Verification items for the finished model (mm, model axes). Face numbers are marked on the shaded views. A direction names the side the tool comes from. Give positions to 0.01 mm unless a question says otherwise; leave off trailing zeros. Write each loop counter-clockwise with the first axis right and the second up, starting at its lowest first coordinate (ties: lowest second). Pieces come first, ordered by that corner, then holes. Notation, with made-up numbers: (81, 51) - (110, 51) arc R28 cw to (110, 83) - close; hole circle Ø4 at (49.5, 42.25). An arc over 180 degrees is marked (long way). Answer as a JSON object with one key per item and string values. Group by question number.
Item 1: Tool access check on the marked faces 1, 2, 3, 4 and 5. Record the directions out of +Z, -Z, +X, -X, +Y, -Y that give a thin tool (end or side, any length) a straight path to the whole face; none if there is none.
Item 2: Sectioned sample at C-C, the plane z = 84. Record the boundary of the cut face in (x, y).
Item 3: Sectioned sample at A-A, the plane y = -46. Record the boundary of the cut face in (x, z), and give its area (3 significant figures).
Item 4: Go/stop test with flat-tipped pins: pin 1 (7.5 mm diameter, centred on x = 35, y = -50, fed in from -Z); pin 2 (5 mm diameter, centred on x = -6.5, z = 36.5, fed in from -Y); pin 3 (3 mm diameter, centred on x = -19.5, y = -58.5, fed in from +Z). Record where each tip stops, or that it passes through.
Item 5: Sectioned sample at D-D, the plane y = -6. Record the boundary of the cut face in (x, z).
Item 6: Draft check along X on the marked faces 6, 7, 8 and 9. Enter one of: +X half, -X half, draft (parallel to the pull), parting line (faces both ways), or undercut.
Item 7: Scan lines: line 1 along X through (y, z) = (-55, 15); line 2 along X through (y, z) = (-12.75, 84); line 3 along Z through (x, y) = (-1, -22.5). Record each from-to range of solid material in increasing order. Write a range as [from, to].
Item 8: Sectioned sample at B-B, the plane x = -3.5. Record the boundary of the cut face in (y, z), and give its area (3 significant figures).
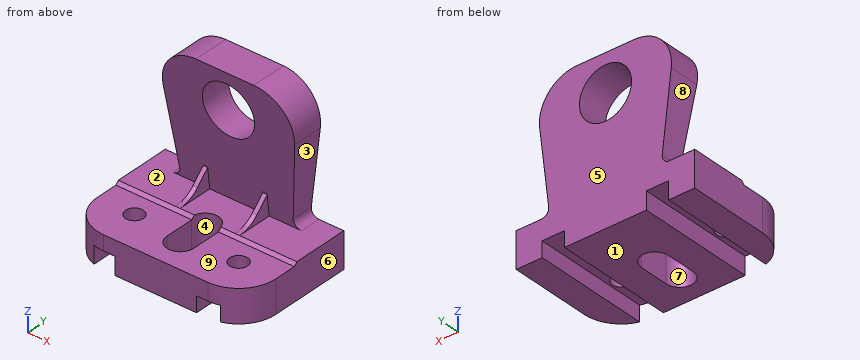
```python
from build123d import *

# Parameters (mm, degrees)
F1_DEPTH      = 60
F2_W          = 15
F2_H          = 11.9018135592
F2_H_2        = 10.3764180094
F3_DEPTH      = 80.001
F5_DEPTH      = 80.001
F6_W          = 3
F6_H          = 15
F7_DEPTH      = 40
F9_DEPTH      = 60.001
F9_DEPTH_BACK = 60.001
F11_D         = 12.1
F13_DEPTH     = 109.001
F15_D         = 35
F16_R         = 25
F17_SIZE      = 1.99999


# Not quite as in the source:
# - a fillet or chamfer is up to 0.001 mm smaller than in the source, because OpenCascade refuses the exact size


with BuildPart() as f1:
    # F0 (on Right) → F1 (new body, symmetric)
    with BuildSketch(Plane.YZ):
        Polygon((-80, 0), (0, 0), (0, 109), (-24, 109), (-14.0000553612, 24), (-40, 24), (-40, 22), (-80, 22), align=None)
    extrude(amount=F1_DEPTH, both=True)

    # F2 (on Front) → F3 (cut, through all)
    with BuildSketch(Plane.XZ):
        with Locations((-35, 5.9509067796)):
            Rectangle(F2_W, F2_H)
        with Locations((35, 5.1882090047)):
            Rectangle(F2_W, F2_H_2)
    extrude(amount=F3_DEPTH, mode=Mode.SUBTRACT)

    # F4 (on Front) → F5 (cut, through all)
    with BuildSketch(Plane.XZ):
        with BuildLine():
            ThreePointArc((-43.1227148243, 24), (-39.3863385559, 25.6774268435), (-38.1569614274, 29.5842030478))
            Line((-38.1569614274, 29.5842030478), (-44.2151375018, 81.0789847612))
            ThreePointArc((-44.2151375018, 81.0789847612), (-38.0682518594, 100.6128657827), (-19.3863705172, 109))
            Line((-19.3863705172, 109), (0, 109))
            Line((0, 109), (19.3863705172, 109))
            ThreePointArc((19.3863705172, 109), (38.0682518594, 100.6128657827), (44.2151375018, 81.0789847612))
            Line((44.2151375018, 81.0789847612), (38.1569614274, 29.5842030478))
            ThreePointArc((38.1569614274, 29.5842030478), (39.3863385559, 25.6774268435), (43.1227148243, 24))
            Line((43.1227148243, 24), (60, 24))
            Line((60, 24), (60, 136.873498559))
            Line((60, 136.873498559), (-60, 136.873498559))
            Line((-60, 136.873498559), (-60, 24))
            Line((-60, 24), (-43.1227148243, 24))
        make_face()
    extrude(amount=F5_DEPTH, mode=Mode.SUBTRACT)

    # F6 (on Front) → F7 (join, through all)
    with BuildSketch(Plane.XZ):
        with Locations((-20, 31.5)):
            Rectangle(F6_W, F6_H)
        with Locations((20, 31.5)):
            Rectangle(F6_W, F6_H)
    extrude(amount=F7_DEPTH)

    # F8 (on Right) → F9 (cut, two sides)
    with BuildSketch(Plane.YZ) as f9_sk:
        with BuildLine():
            Line((-23.8578643763, 29.8578643763), (-15.6543285765, 38.061400176))
            Line((-15.6543285765, 38.061400176), (-16.3282091593, 43.7894168409))
            Line((-16.3282091593, 43.7894168409), (-43.991163373, 43.7894168409))
            Line((-43.991163373, 43.7894168409), (-43.991163373, 24))
            Line((-43.991163373, 24), (-38, 24))
            ThreePointArc((-38, 24), (-30.3463313527, 25.5224093498), (-23.8578643763, 29.8578643763))
        make_face()
    extrude(amount=-F9_DEPTH, mode=Mode.SUBTRACT)
    extrude(f9_sk.sketch, amount=F9_DEPTH_BACK, mode=Mode.SUBTRACT)

    # F11 (through all)
    with Locations(Plane(origin=(0, 0, 0), x_dir=(1, 0, 0), z_dir=(0, 0, -1))):
        with Locations((-35, 55), (35, 55)):
            Hole(F11_D / 2)

    # F12 (on Top) → F13 (cut, through all)
    with BuildSketch(Plane.XY):
        with BuildLine():
            Line((-9, -40), (-9, -60))
            ThreePointArc((-9, -60), (0, -69), (9, -60))
            Line((9, -60), (9, -40))
            ThreePointArc((9, -40), (0, -31), (-9, -40))
        make_face()
    extrude(amount=F13_DEPTH, mode=Mode.SUBTRACT)

    # F15 (through all)
    with Locations(Plane(origin=(0, 0, 0), x_dir=(1, 0, 0), z_dir=(0, 1, 0))):
        with Locations((0, -84)):
            Hole(F15_D / 2)

    # F16
    f16_edges = [f1.edges().sort_by_distance(p)[0] for p in [
        (-60, -80, 11),
        (60, -80, 11),
    ]]
    fillet(f16_edges, radius=F16_R)

    # F17 (size 2 in the source; OpenCascade refuses exactly that, so slightly less here)
    f17_edges = [f1.edges().sort_by_distance(p)[0] for p in [
        (34.5, -40, 24),
        (-34.5, -40, 24),
    ]]
    chamfer(f17_edges, length=F17_SIZE)


solid = f1.part
```
Geometry check:
{
 "1": {"face 1": "-Z, +X, -X, +Y, -Y", "face 2": "-X, -Y", "face 3": "+X, +Y, -Y", "face 4": "+Z, -Z", "face 5": "+Z, -Z, +X, -X, +Y"},
 "2": {"outline": "(-44.39, -21.06) - (-17.5, -21.06) - (-17.5, 0) - (-44.39, 0) - close; (17.5, -21.06) - (44.39, -21.06) - (44.39, 0) - (17.5, 0) - close"},
 "3": {"outline": "(-60, 0) - (-42.5, 0) - (-42.5, 11.9) - (-27.5, 11.9) - (-27.5, 0) - (-9, 0) - (-9, 22) - (-60, 22) - close; (9, 0) - (27.5, 0) - (27.5, 10.38) - (42.5, 10.38) - (42.5, 0) - (60, 0) - (60, 22) - (9, 22) - close", "area": "1,910 mm^2"},
 "4": {"pin 1": "z = 10.38", "pin 2": "y = -15.76", "pin 3": "z = 22"},
 "5": {"outline": "(-60, 0) - (-42.5, 0) - (-42.5, 11.9) - (-27.5, 11.9) - (-27.5, 0) - (27.5, 0) - (27.5, 10.38) - (42.5, 10.38) - (42.5, 0) - (60, 0) - (60, 24) - (43.12, 24) arc R5 cw to (38.16, 29.58) - (44.22, 81.08) arc R25 ccw to (19.39, 109) - (-19.39, 109) arc R25 ccw to (-44.22, 81.08) - (-38.16, 29.58) arc R5 cw to (-43.12, 24) - (-60, 24) - close; hole circle Ø35 at (0, 84)"},
 "6": {"face 6": "+X half", "face 7": "undercut", "face 8": "-X half", "face 9": "draft"},
 "7": {"line 1": "[-60, -41.05], [-28.95, -9], [9, 28.95], [41.05, 60]", "line 2": "[-44.39, -17.5], [17.5, 44.39]", "line 3": "[0, 24], [101.47, 109]"},
 "8": {"outline": "(-80, 0) - (-68.29, 0) - (-68.29, 22) - (-80, 22) - close; (-31.71, 0) - (0, 0) - (0, 66.85) - (-19.04, 66.85) - (-14, 24) - (-31.71, 24) - close; (-24, 109) - (-23.08, 101.15) - (0, 101.15) - (0, 109) - close", "area": "1,910 mm^2"}
}
